Geometry check sheet. Reference: drawing and pictorial views, mm from the part's lowest x, y, z. Round coordinates to 2 decimals unless told otherwise and drop trailing zeros. Loops run counter-clockwise (first coordinate to the right, second up) from the corner with the lowest first, then second, coordinate; pieces in that order, holes last. Notation, with made-up numbers: (-22.75, 81.5) - (-16.75, 81.5) arc R24 cw to (-16.75, 111.5) - close; hole circle Ø10 at (-28.5, 9.25). An arc over 180 degrees is marked (long way). Return JSON: item names as keys, results as strings.
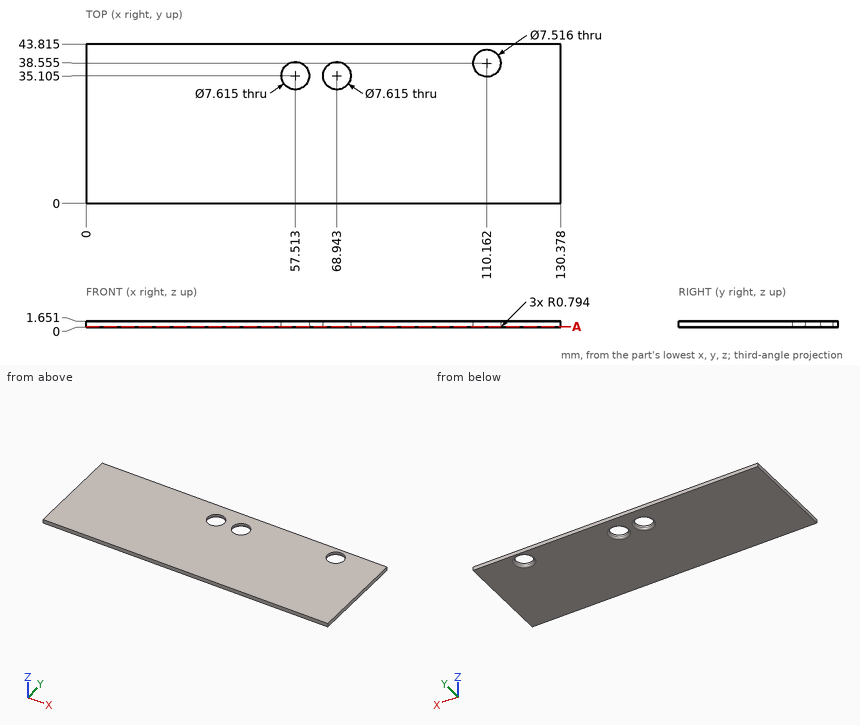
Q1. Sectioned sample at A-A (z = 0.25). Enter the section's corners in (x, y) (1 decimal), plus the area to 3 significant figures.
Answer key:
{"outline": "(0, 0) - (130.4, 0) - (130.4, 43.8) - (0, 43.8) - close; hole circle Ø8 at (57.5, 35.1); hole circle Ø8 at (68.9, 35.1); hole circle Ø7.9 at (110.2, 38.6)", "area": "5,560 mm²"}
Q2. Scan lines: probe 1 along Y at (x, z) = (68.5, 1.3) (1 decimal); probe 2 along X at (y, z) = (40, 1.35); probe 3 along Y at (x, z) = (60, 0.3) (1 decimal). Record each from-to range of solid material in increasing order. Write a range as [from, to].
Answer key:
{"probe 1": "y = [0, 31.3], [38.9, 43.8]", "probe 2": "x = [0, 106.69], [113.63, 130.38]", "probe 3": "y = [0, 32], [38.2, 43.8]"}
Q3. Depth check by flat-ended pin: P1, Ø12, axis at x = 68.94, y = 35.1, coming from the -Z side; P2, Ø6, axis at x = 57.51, y = 35.1, coming from the -Z side. Enter the tip coordinate at first touch or a pass-through.
Answer key:
{"P1": "stops at z = 0", "P2": "passes through"}
